```python
from build123d import *

# Parameters (mm, degrees)
SKETCH_1_W               = 210
SKETCH_1_H               = 190
EXTRUDE_1_DEPTH          = 8
EXTRUDE_2_DEPTH          = 50
SKETCH_3_W               = 20
SKETCH_3_H               = 20
EXTRUDE_3_DEPTH          = 15
SKETCH_8_R               = 4.55
CUT_EXTRUDE_1_DEPTH      = 25
SKETCH_9_W               = 120
SKETCH_9_H               = 100
EXTRUDE_4_DEPTH          = 12
SKETCH_10_R              = 15
CUT_EXTRUDE_2_DEPTH      = 147.608321728
SKETCH_13_R              = 4.55
CUT_EXTRUDE_3_DEPTH      = 154.016338997
PATTERN_CIRCULAR_2_COUNT = 4
SKETCH_14_W              = 120
SKETCH_14_H              = 100
CUT_EXTRUDE_4_DEPTH      = 6
SKETCH_15_W              = 68
SKETCH_15_H              = 76
EXTRUDE_5_DEPTH          = 5
SKETCH_16_W              = 60
SKETCH_16_H              = 60
CUT_EXTRUDE_5_DEPTH      = 5
SKETCH_17_R              = 4.55
CUT_EXTRUDE_6_DEPTH      = 154.016338997
SKETCH_18_W              = 40
SKETCH_18_H              = 20
CUT_EXTRUDE_7_DEPTH      = 6


with BuildPart() as part:
    # 스케치1 → 보스-돌출1 (new body)
    with BuildSketch(Plane.XY):
        Rectangle(SKETCH_1_W, SKETCH_1_H)
    extrude(amount=EXTRUDE_1_DEPTH)

    # 스케치2 → 보스-돌출2 (add)
    with BuildSketch(Plane(origin=(0, 0, 0), x_dir=(-1, 0, 0), z_dir=(0, 0, -1))):
        Polygon((-105, 95), (105, 95), (105, -95), (-105, -95), (-105, -87), (97, -87), (97, 87), (-105, 87), align=None)
    extrude(amount=EXTRUDE_2_DEPTH)

    # 스케치3 → 보스-돌출3 (add)
    with BuildSketch(Plane(origin=(105, 0, 0), x_dir=(0, 0, -1), z_dir=(1, 0, 0))):
        with Locations((10, 77)):
            Rectangle(SKETCH_3_W, SKETCH_3_H)
    extrude_3 = extrude(amount=-EXTRUDE_3_DEPTH)

    # 스케치8 → 컷-돌출1 (cut)
    with BuildSketch(Plane(origin=(105, 0, 0), x_dir=(0, 0, -1), z_dir=(1, 0, 0))):
        with Locations(Location((10, 77, 0), (0, 0, 90))):
            Circle(SKETCH_8_R)
    cut_extrude_1 = extrude(amount=-CUT_EXTRUDE_1_DEPTH, mode=Mode.SUBTRACT)

    # 대칭 복사1: 보스-돌출3, 컷-돌출1 across plane
    add(extrude_3.mirror(Plane(origin=(0, 0, 0), x_dir=(0, 0, 1), z_dir=(0, -1, 0))))
    add(cut_extrude_1.mirror(Plane(origin=(0, 0, 0), x_dir=(0, 0, 1), z_dir=(0, -1, 0))), mode=Mode.SUBTRACT)

    # 스케치9 → 보스-돌출4 (add)
    with BuildSketch(Plane(origin=(0, 0, 0), x_dir=(-1, 0, 0), z_dir=(0, 0, -1))):
        with Locations((37, -37)):
            Rectangle(SKETCH_9_W, SKETCH_9_H)
    extrude(amount=EXTRUDE_4_DEPTH)

    # 스케치10 → 컷-돌출2 (cut, through all)
    with BuildSketch(Plane(origin=(0, 0, -12), x_dir=(-1, 0, 0), z_dir=(0, 0, -1))):
        with Locations((37, -37)):
            Circle(SKETCH_10_R)
    extrude(amount=-CUT_EXTRUDE_2_DEPTH, mode=Mode.SUBTRACT)

    # 스케치13 → 컷-돌출3 (cut, through all)
    with BuildSketch(Plane.XY.offset(8)):
        with Locations((-47, -7)):
            Circle(SKETCH_13_R)
        with Locations((-27, -7)):
            Circle(SKETCH_13_R)
    cut_extrude_3 = extrude(amount=-CUT_EXTRUDE_3_DEPTH, mode=Mode.SUBTRACT)

    # 원형 패턴2: 컷-돌출3 ×4 about axis
    pattern_circular_2_axis = Axis((-37, -37, 0), (0, 0, 1))
    for i in range(1, PATTERN_CIRCULAR_2_COUNT):
        add(cut_extrude_3.rotate(pattern_circular_2_axis, i * 360 / PATTERN_CIRCULAR_2_COUNT), mode=Mode.SUBTRACT)

    # 스케치14 → 컷-돌출4 (cut)
    with BuildSketch(Plane(origin=(0, 0, -12), x_dir=(-1, 0, 0), z_dir=(0, 0, -1))):
        with Locations((37, -37)):
            Rectangle(SKETCH_14_W, SKETCH_14_H)
    extrude(amount=-CUT_EXTRUDE_4_DEPTH, mode=Mode.SUBTRACT)

    # 스케치15 → 보스-돌출5 (add)
    with BuildSketch(Plane(origin=(0, 0, 0), x_dir=(-1, 0, 0), z_dir=(0, 0, -1))):
        with Locations((-71, 30)):
            Rectangle(SKETCH_15_W, SKETCH_15_H)
    extrude(amount=EXTRUDE_5_DEPTH)

    # 스케치16 → 컷-돌출5 (cut)
    with BuildSketch(Plane.XY.offset(8)):
        with Locations((75, 30)):
            Rectangle(SKETCH_16_W, SKETCH_16_H)
    extrude(amount=-CUT_EXTRUDE_5_DEPTH, mode=Mode.SUBTRACT)

    # 스케치17 → 컷-돌출6 (cut, through all)
    with BuildSketch(Plane.XY.offset(8)):
        with Locations((1, 5.05)):
            Circle(SKETCH_17_R)
        with Locations((-80, 5.05)):
            Circle(SKETCH_17_R)
        with Locations((-80, 55.05)):
            Circle(SKETCH_17_R)
        with Locations((1, 55.05)):
            Circle(SKETCH_17_R)
    extrude(amount=-CUT_EXTRUDE_6_DEPTH, mode=Mode.SUBTRACT)

    # 스케치18 → 컷-돌출7 (cut)
    with BuildSketch(Plane(origin=(0, 0, -6), x_dir=(-1, 0, 0), z_dir=(0, 0, -1))):
        with Locations((-3, 3)):
            Rectangle(SKETCH_18_W, SKETCH_18_H)
        with Locations((77, 3)):
            Rectangle(SKETCH_18_W, SKETCH_18_H)
    extrude(amount=-CUT_EXTRUDE_7_DEPTH, mode=Mode.SUBTRACT)


solid = part.part
```
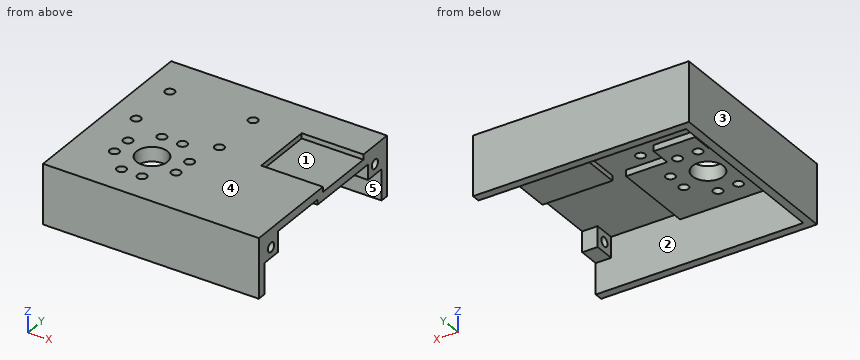
CAD build for the part. Positions are in the model's coordinates, mm. Face numbers are marked on the shaded views. A direction names the side the tool comes from. Coordinates: 2 decimals unless noted, no trailing zeros. Write each loop counter-clockwise with the first axis right and the second up, starting at its lowest first coordinate (ties: lowest second). Pieces come first, ordered by that corner, then holes.
(1) Cut at C-C, the plane y = 5.05. List the corners of the cut face in (x, z).
(2) Drill centre lines: probe 1 along Y at (x, z) = (-80, 4.75); probe 2 along Y at (x, z) = (-67, -2); probe 3 along Y at (x, z) = (92.5, -10.5). Where is each one in solid material? Low to high.
(3) Cut at A-A, the plane y = -77. List the corners of the cut face in (x, z), and give its area (3 significant figures).
(4) Cut at B-B, the plane z = -10. List the corners of the cut face in (x, y).
(5) Flat gauge pins, fed straight in: pin 1 (5.5 mm diameter, centred on y = 77, z = -10, fed in from +X); pin 2 (10.5 mm diameter, centred on x = -47, y = -67, fed in from -Z); pin 3 (16.5 mm diameter, centred on x = 97, y = 74.5, fed in from -Z); pin 4 (10.5 mm diameter, centred on x = -27, y = -7, fed in from +Z). Where does each tip first touch, or does it go through?
(6) Two-plate mould, pull along X, no slides. Class the marked faces 1, 2 and 3: +X half, -X half, draft (parallel to the pull), parting line (faces both ways), or undercut.
(7) Cut at D-D, the plane x = -67. List the corners of the cut face in (y, z).
(8) 3-axis set-ups, long thin cutter, end or side, ignore diameter. For the marked faces 4 and 5: which of +Z, -Z, +X, -X, +Y, -Y reach the whole face in a straight line?
Geometry says:
1. outline: (-105, -50) - (-97, -50) - (-97, 0) - (-84.55, 0) - (-84.55, 8) - (-105, 8) - close; (-75.45, 0) - (-57, 0) - (-57, -6) - (-17, -6) - (-17, 0) - (-3.55, 0) - (-3.55, 8) - (-75.45, 8) - close; (5.55, 0) - (37, 0) - (37, -5) - (105, -5) - (105, 3) - (45, 3) - (45, 8) - (5.55, 8) - close
2. probe 1: y = -95 to 0.5, 9.6 to 50.5, 59.6 to 95
2. probe 2: y = -95 to -51.55, -42.45 to -31.55, -22.45 to -7, 87 to 95
2. probe 3: y = -95 to -81.52, -72.48 to -67, 67 to 72.48, 81.52 to 95
3. outline: (-105, -50) - (-97, -50) - (-97, -6) - (23, -6) - (23, 0) - (90, 0) - (90, -5.45) - (105, -5.45) - (105, 8) - (-105, 8) - close; (90, -20) - (105, -20) - (105, -14.55) - (90, -14.55) - close
3. area: 2,960 mm2
4. outline: (-105, -95) - (105, -95) - (105, -81.55) - (90, -81.55) - (90, -87) - (-97, -87) - (-97, 87) - (90, 87) - (90, 81.55) - (105, 81.55) - (105, 95) - (-105, 95) - close; (90, -72.45) - (105, -72.45) - (105, -67) - (90, -67) - close; (90, 67) - (105, 67) - (105, 72.45) - (90, 72.45) - close
5. pin 1: stops at x = -97
5. pin 2: stops at z = -6
5. pin 3: stops at z = -20
5. pin 4: stops at z = 8
6. face 1: draft
6. face 2: undercut
6. face 3: -X half
7. outline: (-95, -50) - (-87, -50) - (-87, -6) - (-51.55, -6) - (-51.55, 8) - (-95, 8) - close; (-42.45, -6) - (-31.55, -6) - (-31.55, 8) - (-42.45, 8) - close; (-22.45, -6) - (-7, -6) - (-7, 0) - (87, 0) - (87, -50) - (95, -50) - (95, 8) - (-22.45, 8) - close
8. face 4: +Z, +X, -X, +Y, -Y
8. face 5: -Z
